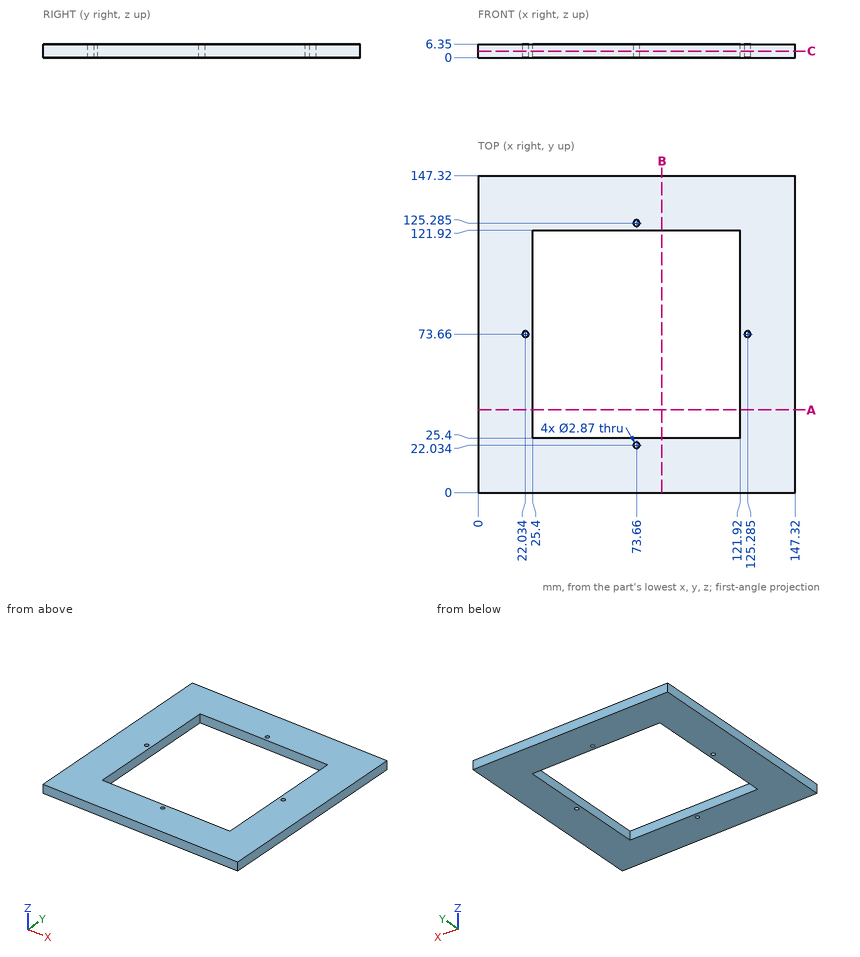
The drawing under review shows one solid part. Ordinate dimensions are in mm from its lowest x, y, z. Coordinates: 2 decimals unless noted, no trailing zeros. Loops run counter-clockwise (first coordinate to the right, second up) from the corner with the lowest first, then second, coordinate; pieces in that order, holes last.
Item 1: Clearance check with a flat-ended pin moving along its axis: pin 1 (1.5 mm diameter, centred on y = 132, z = 5, fed in from -X). State where the tip first meets the part, or that it passes through.
Completed:
pin 1: stops at x = 0
Item 2: Add section C-C (z = 3). Write out the cut boundary in (x, y) (1 decimal).
Completed:
outline: (0, 0) - (147.3, 0) - (147.3, 147.3) - (0, 147.3) - close; hole circle Ø2.9 at (22, 73.7); hole (25.4, 25.4) - (121.9, 25.4) - (121.9, 121.9) - (25.4, 121.9) - close; hole circle Ø2.9 at (73.7, 22); hole circle Ø2.9 at (73.7, 125.3); hole circle Ø2.9 at (125.3, 73.7)
Item 3: Add section A-A (y = 38.5). Write out the cut boundary in (x, z).
Completed:
outline: (0, 0) - (25.4, 0) - (25.4, 6.35) - (0, 6.35) - close; (121.92, 0) - (147.32, 0) - (147.32, 6.35) - (121.92, 6.35) - close
Item 4: Wall thickness on L1, parallel to X at y = 73.66, z = 5; L2, parallel to Y at x = 95.5, z = 2.25: over which ranges is each line inside the solid? List them lowest first.
Completed:
L1: x = 0 to 20.6, 23.47 to 25.4, 121.92 to 123.85, 126.72 to 147.32
L2: y = 0 to 25.4, 121.92 to 147.32
